CAD build for the part. Positions are in the model's coordinates, mm. A direction names the side the tool comes from. Round coordinates to 2 decimals unless told otherwise and drop trailing zeros. Write each loop counter-clockwise with the first axis right and the second up, starting at its lowest first coordinate (ties: lowest second). Pieces come first, ordered by that corner, then holes. Notation, with made-up numbers: (57.25, 48.5) - (88.25, 48.5) arc R20 ccw to (88.25, 53.5) - close; hole circle Ø7 at (26, 67). An arc over 180 degrees is marked (long way). Put each result on its own line as item: value. Start each with the question number.
Item 1: Cut at C-C (z = 47.5). Give the cut face in (x, y), and give its area (3 significant figures).
Item 2: Pin check, flat tips, straight feed: pin 1 Ø4 at (x, z) = (-20.5, 18) entering from +Y; pin 2 Ø12 at (x, z) = (13, 42) entering from -Y; pin 3 Ø8 at (x, y) = (38, -40) entering from +Z; pin 4 Ø4 at (x, z) = (-11, 32.5) entering from +Y. Stop position of each tip, or through.
Item 3: Mould opens along X. For faces 1 (the flat face through (-29.919, -12, 2)), 2 (the flat face through (10, -11, 5)), 3 (the flat face through (1, 16, 5)), 4 (the cylindrical face through (-17.89, -9.83, 37.04)) say: released by +X, released by -X, zero draft, split by the parting line, or undercut.
Item 4: Drill centre lines: line 1 (X direction, y = -11.5, z = 36.5); line 2 (Y direction, x = 10, z = 63); line 3 (Z direction, x = -22.5, y = -13). Where is each one in solid material? Low to high. Write a range as from..to.
Item 5: Cut at D-D (x = -21). Give the cut face in (y, z).
Item 6: 3-axis set-ups, long thin cutter, end or side, ignore diameter. For faces 5 (the flat face through (10, -10, 0)), 6 (the cylindrical face through (-10.55, -26.88, 37.04)): which of +Z, -Z, +X, -X, +Y, -Y reach the whole face in a straight line?
Item 7: Cut at A-A (x = 6). Give the cut face in (y, z).
Item 8: Cut at B-B (y = -1). Give the cut face in (x, z).
```python
from build123d import *

# Parameters (mm, degrees)
SKETCH1_W           = 80
SKETCH1_H           = 80
BOSS_EXTRUDE1_DEPTH = 5
SKETCH2_R           = 28
SKETCH2_R_2         = 26
EXTRUDE_THIN1_DEPTH = 65


with BuildPart() as part:
    # Sketch1 → Boss-Extrude1 (new body)
    with BuildSketch(Plane.XY):
        with Locations((10.081300813, -11.056910569)):
            Rectangle(SKETCH1_W, SKETCH1_H)
    extrude(amount=BOSS_EXTRUDE1_DEPTH)

    # Sketch2 → Extrude-Thin1 (add)
    with BuildSketch(Plane.XY.offset(5)):
        with Locations((10.081300813, -11.056910569)):
            Circle(SKETCH2_R)
        with Locations((10.081300813, -11.056910569)):
            Circle(SKETCH2_R_2, mode=Mode.SUBTRACT)
    extrude(amount=EXTRUDE_THIN1_DEPTH)


solid = part.part
```
Output values:
1. outline: circle Ø56 at (10.08, -11.06); hole circle Ø52 at (10.08, -11.06)
1. area: 339 mm2
2. pin 1: through
2. pin 2: y = -39.06
2. pin 3: z = 5
2. pin 4: y = 9.43
3. face 1: released by -X
3. face 2: undercut
3. face 3: zero draft
3. face 4: split by the parting line
4. line 1: -17.92..-15.91, 36.08..38.08
4. line 2: -39.06..-37.06, 14.94..16.94
4. line 3: 0..5
5. outline: (-51.06, 0) - (28.94, 0) - (28.94, 5) - (-51.06, 5) - close
6. face 5: -Z, +X, -X, +Y, -Y
6. face 6: +Z
7. outline: (-51.06, 0) - (28.94, 0) - (28.94, 5) - (16.64, 5) - (16.64, 70) - (14.62, 70) - (14.62, 5) - (-36.73, 5) - (-36.73, 70) - (-38.76, 70) - (-38.76, 5) - (-51.06, 5) - close
8. outline: (-29.92, 0) - (50.08, 0) - (50.08, 5) - (36.21, 5) - (36.21, 70) - (34.06, 70) - (34.06, 5) - (-13.89, 5) - (-13.89, 70) - (-16.05, 70) - (-16.05, 5) - (-29.92, 5) - close
